Input: dimensioned drawing with shaded views. Units: mm. Origin: part minimum x, y, z. Round coordinates to 2 decimals unless told otherwise and drop trailing zeros. Loops run counter-clockwise (first coordinate to the right, second up) from the corner with the lowest first, then second, coordinate; pieces in that order, holes last. Notation, with made-up numbers: (87.25, 28) -> (99.25, 28) arc R21 ccw to (99.25, 42) -> close; hole circle Ø7 at (-21.5, -9). An arc over 180 degrees is marked (long way). Answer as a JSON object with one key per item and string values.
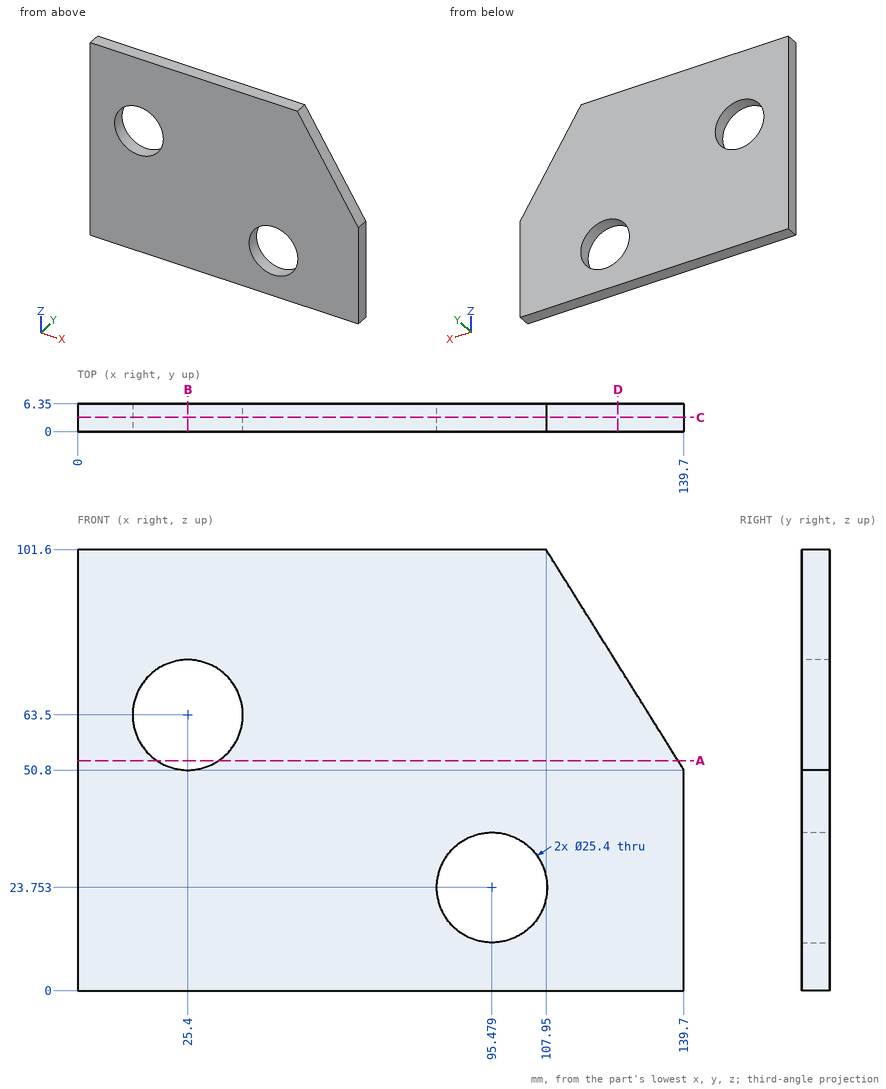
1) Section A-A, the plane z = 53. Output: boundary loops of the cut face in (x, y) (3 decimals).
Output:
{"outline": "(0, 0) -> (18.256, 0) -> (18.256, 6.35) -> (0, 6.35) -> close; (32.544, 0) -> (138.325, 0) -> (138.325, 6.35) -> (32.544, 6.35) -> close"}
2) Section D-D, the plane x = 124.5. Output: boundary loops of the cut face in (y, z).
Output:
{"outline": "(0, 0) -> (6.35, 0) -> (6.35, 75.12) -> (0, 75.12) -> close"}
3) Contact query for a flat-ended pin moving along its axis: P1, Ø23, axis at x = 95.48, z = 23.75, coming from the -Y side. Output: stop coordinate, or through.
Output:
{"P1": "passes through"}
4) Section B-B, the plane x = 25.4. Output: boundary loops of the cut face in (y, z).
Output:
{"outline": "(0, 0) -> (6.35, 0) -> (6.35, 50.8) -> (0, 50.8) -> close; (0, 76.2) -> (6.35, 76.2) -> (6.35, 101.6) -> (0, 101.6) -> close"}
5) Section C-C, the plane y = 3.25. Output: boundary loops of the cut face in (x, z), plus the area to 3 significant figures.
Output:
{"outline": "(0, 0) -> (139.7, 0) -> (139.7, 50.8) -> (107.95, 101.6) -> (0, 101.6) -> close; hole circle Ø25.4 at (25.4, 63.5); hole circle Ø25.4 at (95.48, 23.75)", "area": "12,400 mm^2"}
6) Ray query, probe 1 along Z at (x, y) = (25.4, 4); probe 2 along X at (y, z) = (1.75, 55) (1 decimal); probe 3 along X at (y, z) = (3.75, 23). Return the intervals inside material, ascending.
Output:
{"probe 1": "z = 0 to 50.8, 76.2 to 101.6", "probe 2": "x = 0 to 16, 34.8 to 137.1", "probe 3": "x = 0 to 82.8, 108.16 to 139.7"}
